from build123d import *

# Parameters (mm, degrees)
M6X1_0_1_D     = 5
M6X1_0_1_DEPTH = 12
M6X1_0_1_TIP   = 1.502151548
CHAMFER_1_SIZE = 0.5


with BuildPart() as part:
    # 스케치1 → 회전1 (revolve)
    with BuildSketch(Plane(origin=(0, 0, 0), x_dir=(0, 0, -1), z_dir=(1, 0, 0))):
        Polygon((0, 0), (0, 5), (14, 5), (16, 3), (16, 2.5), (60, 2.5), (60, 0), align=None)
    revolve(axis=Axis((0, 0, -60), (0, 0, 1)))

    # M6x1.0 나사 구멍1
    with Locations(Plane.XY):
        with Locations((0, 0)):
            Hole(M6X1_0_1_D / 2, depth=M6X1_0_1_DEPTH)
            with Locations((0, 0, -(M6X1_0_1_DEPTH + M6X1_0_1_TIP / 2))):  # 118° drill point
                Cone(0, M6X1_0_1_D / 2, M6X1_0_1_TIP, mode=Mode.SUBTRACT)

    # 모따기1
    chamfer_1_edges = [part.edges().sort_by_distance(p)[0] for p in [
        (0, -2.5, -60),
    ]]
    chamfer(chamfer_1_edges, length=CHAMFER_1_SIZE)


solid = part.part
CAD build for the part. Positions are in the model's coordinates, mm. A direction names the side the tool comes from. Round coordinates to 2 decimals unless told otherwise and drop trailing zeros. Write each loop counter-clockwise with the first axis right and the second up, starting at its lowest first coordinate (ties: lowest second). Pieces come first, ordered by that corner, then holes. Notation, with made-up numbers: (58.25, 44) -> (109.25, 44) arc R27 cw to (109.25, 61) -> close; hole circle Ø8 at (-32, 22). An arc over 180 degrees is marked (long way). Answer as a JSON object with one key per item and string values.
(1) Two-plate mould, pull along Y, no slides. Class faces 4 (the face through (-0.094, -0.424, -13.241)), 5 (the face through (-2, -2, -16)), 6 (the face through (4.88, -1.08, -7.1)): +Y half, -Y half, draft (parallel to the pull), parting line (faces both ways), or undercut.
Reported:
{"face 4": "undercut", "face 5": "draft", "face 6": "parting line"}
(2) Band-saw the part on A-A, the plane z = -8. List the corners of the cut face in (x, y).
Reported:
{"outline": "circle Ø10 at (0, 0); hole circle Ø5 at (0, 0)"}
(3) Probe probe 1 along Y at (x, z) = (0, -9.25); probe 2 along X at (y, z) = (-4, -6). List the from-to ranges inside material, lowest first. Write a range as [from, to].
Reported:
{"probe 1": "y = [-5, -2.5], [2.5, 5]", "probe 2": "x = [-3, 3]"}
(4) Pin check, flat tips, straight feed: P1, Ø1, axis at x = -3, y = -3, coming from the -Z side; P2, Ø1.5, axis at y = 0, z = -30.5, coming from the -X side; P3, Ø4, axis at x = -3, y = 3, coming from the -Z side. Stop position of each tip, or through.
Reported:
{"P1": "stops at z = -15.26", "P2": "stops at x = -2.5", "P3": "stops at z = -59.76"}
(5) Band-saw the part on B-B, the plane z = -28.5. List the corners of the cut face in (x, y), then the cut area to 3 significant figures.
Reported:
{"outline": "circle Ø5 at (0, 0)", "area": "19.6 mm^2"}
(6) Which spindle directions (+Z, -Z, +X, -X, +Y, -Y) get a long thin tool onto all of the face, cutting with end or side? Do faces 1 (the face through (0, 0, -60)), 2 (the face through (2.44, -0.54, -38.05)), 3 (the face through (0.54, -2.44, -6.08)). Say none if no direction does.
Reported:
{"face 1": "-Z, +X, -X, +Y, -Y", "face 2": "-Z", "face 3": "+Z"}
